```python
from build123d import *

# Parameters (mm, degrees)
BOSS_EXTRUDE1_DEPTH = 40
SKETCH2_R           = 2.991229743
CUT_EXTRUDE1_DEPTH  = 21
SKETCH3_R           = 1.664454023
CUT_EXTRUDE2_DEPTH  = 40


with BuildPart() as part:
    # Sketch1 → Boss-Extrude1 (new body)
    with BuildSketch(Plane.XY):
        Polygon((12.727272727, -8.568181818), (14.727272727, -8.568181818), (14.727272727, 3.431818182), (-5.272727273, 3.431818182), (-5.272727273, -6.568181818), (-8.272727273, -6.568181818), (-8.272727273, -8.568181818), (2.727272727, -8.568181818), (2.727272727, -6.568181818), (12.727272727, -6.568181818), align=None)
    extrude(amount=BOSS_EXTRUDE1_DEPTH)

    # Sketch2 → Cut-Extrude1 (cut, through all)
    with BuildSketch(Plane.ZY.offset(5.272727273)):
        with Locations((4, -0.568181818)):
            Circle(SKETCH2_R)
        with Locations((36, -0.568181818)):
            Circle(SKETCH2_R)
    extrude(amount=-CUT_EXTRUDE1_DEPTH, mode=Mode.SUBTRACT)

    # Sketch3 → Cut-Extrude2 (cut)
    with BuildSketch(Plane(origin=(0, 3.431818182, 0), x_dir=(1, 0, 0), z_dir=(0, 1, 0))):
        with Locations((7.727272727, -30)):
            Circle(SKETCH3_R)
        with Locations((7.727272727, -10)):
            Circle(SKETCH3_R)
    extrude(amount=-CUT_EXTRUDE2_DEPTH, mode=Mode.SUBTRACT)


solid = part.part
```
Work out the finished part from the listing and answer in its coordinate system (mm). A direction names the side the tool comes from. Coordinates: 2 decimals unless noted, no trailing zeros. Order: outer loops, then holes, each group sorted by start corner. A loop starts at its lowest first (then second) coordinate and runs counter-clockwise, first axis right, second up. Notation, with made-up numbers: M -4,55 L 32,55 A11 ccw 32,71 Z; hole C -29.75,4.5 d1. An arc over 180 degrees is marked long. Use CSV: the item, a comma, the result in double quotes.
1) Section D-D on y = -5 is taken. Write down the section's boundary in (x, z).
Worked out:
outline,"M -5.27,0 L 14.73,0 L 14.73,40 L -5.27,40 Z; hole C 7.73,10 d3.33; hole C 7.73,30 d3.33"
2) Flat-ended cylindrical pins translate along their axes: pin 1 Ø2 at (x, z) = (7.73, 30) entering from +Y; pin 2 Ø4 at (x, z) = (7.73, 10) entering from -Y; pin 3 Ø3 at (y, z) = (1, 14) entering from -X. Find the tip coordinate at first contact, or state that the pin passes through.
Worked out:
pin 1,"passes through"
pin 2,"stops at y = -6.57"
pin 3,"stops at x = -5.27"
3) Section C-C on z = 30 is taken. Write down the section's boundary in (x, y).
Worked out:
outline,"M -8.27,-8.57 L 2.73,-8.57 L 2.73,-6.57 L 6.06,-6.57 L 6.06,3.43 L -5.27,3.43 L -5.27,-6.57 L -8.27,-6.57 Z; M 9.39,-6.57 L 12.73,-6.57 L 12.73,-8.57 L 14.73,-8.57 L 14.73,3.43 L 9.39,3.43 Z"
4) Section A-A on y = 1.75 is taken. Write down the section's boundary in (x, z), plus the area to 3 significant figures.
Worked out:
outline,"M -5.27,0 L 14.73,0 L 14.73,2.11 L -5.27,2.11 Z; M -5.27,5.89 L 14.73,5.89 L 14.73,34.11 L -5.27,34.11 Z; M -5.27,37.89 L 14.73,37.89 L 14.73,40 L -5.27,40 Z; hole C 7.73,10 d3.33; hole C 7.73,30 d3.33"
area,"631 mm^2"
5) Determine the mould class of faces 1 (the face through (2.727, -8, 20)), 2 (the face through (14, -8.568, 20)), 3 (the face through (-8.273, -8, 20)), 4 (the face through (8, -6.568, 20)) for opening direction X: released by +X, released by -X, zero draft, split by the parting line, or undercut.
Worked out:
face 1,"undercut"
face 2,"zero draft"
face 3,"released by -X"
face 4,"undercut"
6) For faces 5 (the face through (-3, -8.568, 20)), 6 (the face through (-5.273, -1, 20)), 7 (the face through (12.727, -8, 20)), determine the directions among +Z, -Z, +X, -X, +Y, -Y from which every point of the face is accessible in a straight line to the end or side of a thin tool.
Worked out:
face 5,"+Z, -Z, +X, -X, -Y"
face 6,"+Z, -Z, -X, +Y"
face 7,"+Z, -Z, -Y"
7) Consider line 1 (Y direction, x = 5, z = 4); line 2 (Z direction, x = 10, y = 1.25); line 3 (X direction, y = -1.5, z = 30). Determine where each line is inside the solid, lowest interval first. Write a range as [from, to].
Worked out:
line 1,"y = [-6.57, -3.56], [2.42, 3.43]"
line 2,"z = [0, 1.62], [6.38, 33.62], [38.38, 40]"
line 3,"x = [-5.27, 6.06], [9.39, 14.73]"
8) Section B-B on x = 8 is taken. Write down the section's boundary in (y, z), plus the area to 3 significant figures.
Worked out:
outline,"M -6.57,0 L 3.43,0 L 3.43,8.36 L -6.57,8.36 Z; M -6.57,11.64 L 3.43,11.64 L 3.43,28.36 L -6.57,28.36 Z; M -6.57,31.64 L 3.43,31.64 L 3.43,40 L -6.57,40 Z; hole C -0.57,4 d5.98; hole C -0.57,36 d5.98"
area,"278 mm^2"
